from build123d import *

# Parameters (mm, degrees)
F0_R     = 20.32
F1_DEPTH = 25.4
F3_DEPTH = 12.7
F4_R     = 9.525
F5_DEPTH = 25.4


with BuildPart() as f1:
    # F0 (on Top) → F1 (new body)
    with BuildSketch(Plane.XY):
        Circle(F0_R)
    extrude(amount=F1_DEPTH)

    # F2 (on face) → F3 (cut)
    with BuildSketch(Plane.XY.offset(25.4)):
        with BuildLine():
            Line((1.27, 14.549678), (0.2032, 17.06759))
            ThreePointArc((0.2032, 17.06759), (0, 17.0688), (-0.2032, 17.06759))
            Line((-0.2032, 17.06759), (-1.27, 14.549678))
            Line((-1.27, 14.549678), (-2.5488, 14.428136))
            Line((-2.5488, 14.428136), (-4.230933, 16.584145))
            ThreePointArc((-4.230933, 16.584145), (-4.427523, 16.532721), (-4.623486, 16.478961))
            Line((-4.623486, 16.478961), (-5.002252, 13.770736))
            Line((-5.002252, 13.770736), (-5.925394, 13.445678))
            Line((-5.925394, 13.445678), (-8.073251, 15.138207))
            ThreePointArc((-8.073251, 15.138207), (-8.2519, 15.041375), (-8.429382, 14.942423))
            Line((-8.429382, 14.942423), (-8.151213, 12.222024))
            Line((-8.151213, 12.222024), (-8.970171, 11.686149))
            Line((-8.970171, 11.686149), (-11.459754, 12.817486))
            ThreePointArc((-11.459754, 12.817486), (-11.610147, 12.680835), (-11.758903, 12.542404))
            Line((-11.758903, 12.542404), (-10.839857, 9.966884))
            Line((-10.839857, 9.966884), (-11.507351, 9.251129))
            Line((-11.507351, 9.251129), (-14.194932, 9.75596))
            ThreePointArc((-14.194932, 9.75596), (-14.308389, 9.58738), (-14.419831, 9.417461))
            Line((-14.419831, 9.417461), (-12.912966, 7.135509))
            Line((-12.912966, 7.135509), (-13.390461, 6.281195))
            Line((-13.390461, 6.281195), (-16.120882, 6.130376))
            ThreePointArc((-16.120882, 6.130376), (-16.190851, 5.939599), (-16.258545, 5.748002))
            Line((-16.258545, 5.748002), (-14.250855, 3.891358))
            Line((-14.250855, 3.891358), (-14.510784, 2.947806))
            Line((-14.510784, 2.947806), (-17.126414, 2.150044))
            ThreePointArc((-17.126414, 2.150044), (-17.148857, 1.948083), (-17.168895, 1.74587))
            Line((-17.168895, 1.74587), (-14.776286, 0.42172))
            Line((-14.776286, 0.42172), (-14.803644, -0.556597))
            Line((-14.803644, -0.556597), (-17.153479, -1.955247))
            ThreePointArc((-17.153479, -1.955247), (-17.1271, -2.156731), (-17.098324, -2.357887))
            Line((-17.098324, -2.357887), (-14.458926, -3.073097))
            Line((-14.458926, -3.073097), (-14.252132, -4.0297))
            Line((-14.252132, -4.0297), (-16.200513, -5.948491))
            ThreePointArc((-16.200513, -5.948491), (-16.126835, -6.137867), (-16.050907, -6.326352))
            Line((-16.050907, -6.326352), (-13.317096, -6.391332))
            Line((-13.317096, -6.391332), (-12.888089, -7.270995))
            Line((-12.888089, -7.270995), (-14.322533, -9.599153))
            ThreePointArc((-14.322533, -9.599153), (-14.205809, -9.765488), (-14.087113, -9.930421))
            Line((-14.087113, -9.930421), (-11.416715, -9.34142))
            Line((-11.416715, -9.34142), (-10.790263, -10.093358))
            Line((-10.790263, -10.093358), (-11.627957, -12.696475))
            ThreePointArc((-11.627957, -12.696475), (-11.474926, -12.830166), (-11.320314, -12.962025))
            Line((-11.320314, -12.962025), (-8.867496, -11.753047))
            Line((-8.867496, -11.753047), (-8.079764, -12.33385))
            Line((-8.079764, -12.33385), (-8.272347, -15.061644))
            ThreePointArc((-8.272347, -15.061644), (-8.091843, -15.154973), (-7.910242, -15.246146))
            Line((-7.910242, -15.246146), (-5.816608, -13.486986))
            Line((-5.816608, -13.486986), (-4.913073, -13.863124))
            Line((-4.913073, -13.863124), (-4.449427, -16.558115))
            ThreePointArc((-4.449427, -16.558115), (-4.251872, -16.605694), (-4.053764, -16.650917))
            Line((-4.053764, -16.650917), (-2.440183, -14.443135))
            Line((-2.440183, -14.443135), (-1.473008, -14.592893))
            Line((-1.473008, -14.592893), (-0.3799, -17.099496))
            ThreePointArc((-0.3799, -17.099496), (-0.176698, -17.098577), (0.026478, -17.09524))
            Line((0.026478, -17.09524), (1.066852, -14.566294))
            Line((1.066852, -14.566294), (2.041831, -14.481025))
            Line((2.041831, -14.481025), (3.701295, -16.654531))
            ThreePointArc((3.701295, -16.654531), (3.898411, -16.605168), (4.094927, -16.553463))
            Line((4.094927, -16.553463), (4.502032, -13.849353))
            Line((4.502032, -13.849353), (5.428527, -13.53398))
            Line((5.428527, -13.53398), (7.558543, -15.248908))
            ThreePointArc((7.558543, -15.248908), (7.738196, -15.153952), (7.916705, -15.056864))
            Line((7.916705, -15.056864), (7.667038, -12.333701))
            Line((7.667038, -12.333701), (8.491563, -11.806432))
            Line((8.491563, -11.806432), (10.969162, -12.963777))
            ThreePointArc((10.969162, -12.963777), (11.120978, -12.828709), (11.271176, -12.691842))
            Line((11.271176, -12.691842), (10.37915, -10.10684))
            Line((10.37915, -10.10684), (11.054103, -9.398114))
            Line((11.054103, -9.398114), (13.73625, -9.931061))
            ThreePointArc((13.73625, -9.931061), (13.851466, -9.763679), (13.964681, -9.594936))
            Line((13.964681, -9.594936), (12.481795, -7.297329))
            Line((12.481795, -7.297329), (12.96821, -6.448063))
            Line((12.96821, -6.448063), (15.700061, -6.325844))
            ThreePointArc((15.700061, -6.325844), (15.772024, -6.13581), (15.84172, -5.944933))
            Line((15.84172, -5.944933), (13.853583, -4.067366))
            Line((13.853583, -4.067366), (14.123378, -3.126588))
            Line((14.123378, -3.126588), (16.747219, -2.356259))
            ThreePointArc((16.747219, -2.356259), (16.771776, -2.154545), (16.793929, -1.952553))
            Line((16.793929, -1.952553), (14.415319, -0.603421))
            Line((14.415319, -0.603421), (14.452919, 0.374556))
            Line((14.452919, 0.374556), (16.817272, 1.748523))
            ThreePointArc((16.817272, 1.748523), (16.793004, 1.950272), (16.766336, 2.151718))
            Line((16.766336, 2.151718), (14.134573, 2.894528))
            Line((14.134573, 2.894528), (13.937808, 3.853244))
            Line((13.937808, 3.853244), (15.906174, 5.751527))
            ThreePointArc((15.906174, 5.751527), (15.834483, 5.941664), (15.760534, 6.130934))
            Line((15.760534, 6.130934), (13.027553, 6.224538))
            Line((13.027553, 6.224538), (12.607782, 7.108646))
            Line((12.607782, 7.108646), (14.066526, 9.421655))
            ThreePointArc((14.066526, 9.421655), (13.95155, 9.589202), (13.834588, 9.75537))
            Line((13.834588, 9.75537), (11.158169, 9.194365))
            Line((11.158169, 9.194365), (10.539626, 9.952822))
            Line((10.539626, 9.952822), (11.404533, 12.547024))
            ThreePointArc((11.404533, 12.547024), (11.25291, 12.68231), (11.099687, 12.815781))
            Line((11.099687, 12.815781), (8.634343, 11.632554))
            Line((8.634343, 11.632554), (7.852737, 12.221575))
            Line((7.852737, 12.221575), (8.073874, 14.947202))
            ThreePointArc((8.073874, 14.947202), (7.894358, 15.042416), (7.713721, 15.135486))
            Line((7.713721, 15.135486), (5.60178, 13.398347))
            Line((5.60178, 13.398347), (4.702234, 13.783926))
            Line((4.702234, 13.783926), (4.266835, 16.483624))
            ThreePointArc((4.266835, 16.483624), (4.069789, 16.533269), (3.872166, 16.580564))
            Line((3.872166, 16.580564), (2.235553, 14.389801))
            Line((2.235553, 14.389801), (1.27, 14.549678))
        make_face()
    extrude(amount=-F3_DEPTH, mode=Mode.SUBTRACT)

    # F4 (on face) → F5 (join)
    with BuildSketch(Plane(origin=(0, 0, 0), x_dir=(1, 0, 0), z_dir=(0, 0, -1))):
        Circle(F4_R)
    extrude(amount=F5_DEPTH)


solid = f1.part
Check sheet for the modelled part. Datum: model origin and axes. Units: mm. Give positions to 0.01 mm unless a question says otherwise; leave off trailing zeros. Loops run counter-clockwise (first coordinate to the right, second up) from the corner with the lowest first, then second, coordinate; pieces in that order, holes last. Notation, with made-up numbers: M 57,83 L 64,83 A10 ccw 64,89 Z; hole C -4.5,-37.75 d8. An arc over 180 degrees is marked long. Answer as a JSON object with one key per item and string values. Group by question number.
Q1. Release check for a two-part mould opening along X. For faces 1 (the flat face through (0, 0, -25.4)), 2 (the flat face through (-15.8, -2.71, 19.14)), 3 (the cylindrical face through (-2.645, 20.147, 12.522)) record: released by +X, released by -X, zero draft, split by the parting line, or undercut.
Q2. Material ranges on line 1 along Z through (x, y) = (1, 0.5); line 2 along Z through (x, y) = (14.5, 1); line 3 along Y through (x, z) = (-1, 18.5), recorded low to high. Write a range as [from, to].
Q3. Go/stop test with flat-tipped pins: P1, Ø3, axis at y = -9.5, z = -15, coming from the -X side; P2, Ø1, axis at x = 2, z = 17.5, coming from the -Y side; P3, Ø4, axis at y = 6.5, z = 8.5, coming from the -X side; P4, Ø2, axis at y = 11, z = -4.5, coming from the +X side. Record where each tip stops, or that it passes through.
Q4. Cross-section at B-B on z = 2.5. Record the cut outline in (x, y).
Q5. Cross-section at A-A on z = -12. Record the cut outline in (x, y) (3 decimals).
Evaluation:
{
 "1": {"face 1": "zero draft", "face 2": "undercut", "face 3": "split by the parting line"},
 "2": {"line 1": "z = [-25.4, 12.7]", "line 2": "z = [0, 12.7]", "line 3": "y = [-20.3, -15.68], [15.19, 20.3]"},
 "3": {"P1": "stops at x = -5.17", "P2": "stops at y = -20.26", "P3": "stops at x = -19.82", "P4": "passes through"},
 "4": {"outline": "C 0,0 d40.64"},
 "5": {"outline": "C 0,0 d19.05"}
}
